Check sheet for the modelled part. Datum: model origin and axes. Units: mm. Coordinates: 2 decimals unless noted, no trailing zeros. Loops run counter-clockwise (first coordinate to the right, second up) from the corner with the lowest first, then second, coordinate; pieces in that order, holes last. Notation, with made-up numbers: (-32, 47) -> (14, 47) arc R7 ccw to (14, 53) -> close; hole circle Ø2 at (-26.5, 83). An arc over 180 degrees is marked (long way). Use one line per item in the form item = value.
from build123d import *

# Parameters (mm, degrees)
SKETCH1_R           = 11.25
SKETCH1_R_2         = 1.75
BOSS_EXTRUDE1_DEPTH = 3


with BuildPart() as part:
    # Sketch1 → Boss-Extrude1 (new body)
    with BuildSketch(Plane.XY):
        with BuildLine():
            Line((-125.662997175, -15.687527708), (-84.162997175, -15.687527708))
            Line((-84.162997175, -15.687527708), (-84.162997175, 25.812472292))
            Line((-84.162997175, 25.812472292), (-84.162997175, 30.812472292))
            Line((-84.162997175, 30.812472292), (-93.033440026, 55.812472292))
            Line((-93.033440026, 55.812472292), (-138.033440026, 55.812472292))
            Line((-138.033440026, 55.812472292), (-138.033440026, 54.312472292))
            ThreePointArc((-138.033440026, 54.312472292), (-126.533440026, 42.812472292), (-138.033440026, 31.312472292))
            Line((-138.033440026, 31.312472292), (-138.033440026, 30.812472292))
            Line((-138.033440026, 30.812472292), (-125.662997175, 30.812472292))
            Line((-125.662997175, 30.812472292), (-125.662997175, 25.812472292))
            Line((-125.662997175, 25.812472292), (-125.662997175, -15.687527708))
        make_face()
        with Locations((-108.033440026, 42.812472292)):
            Circle(SKETCH1_R, mode=Mode.SUBTRACT)
        with Locations((-89.412997175, 20.562472292)):
            Circle(SKETCH1_R_2, mode=Mode.SUBTRACT)
        with Locations((-120.412997175, 20.562472292)):
            Circle(SKETCH1_R_2, mode=Mode.SUBTRACT)
        with Locations((-120.412997175, -10.437527708)):
            Circle(SKETCH1_R_2, mode=Mode.SUBTRACT)
        with Locations((-89.412997175, -10.437527708)):
            Circle(SKETCH1_R_2, mode=Mode.SUBTRACT)
        with Locations((-122.733440026, 50.812472292)):
            Circle(SKETCH1_R_2, mode=Mode.SUBTRACT)
        with Locations((-122.733440026, 33.812472292)):
            Circle(SKETCH1_R_2, mode=Mode.SUBTRACT)
        with Locations((-92.733440026, 33.812472292)):
            Circle(SKETCH1_R_2, mode=Mode.SUBTRACT)
    extrude(amount=BOSS_EXTRUDE1_DEPTH)


solid = part.part
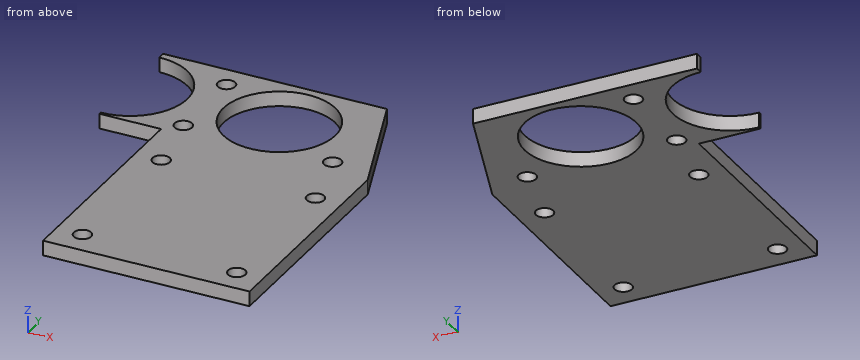
(1) Section check C-C, the plane z = 2.35. Give the number of separate pieces and of enclosed holes in the cut face, plus the area to 3 significant figures.
Established:
separate_pieces = 1
enclosed_holes = 8
area = 2,490 mm²
(2) Go/stop test with a flat-tipped pin: P1, Ø1, axis at y = 34, z = 2.5, coming from the +X side. Record where the tip stops, or that it passes through.
Established:
P1 = -85.12
(3) Section check A-A, the plane x = -105. Record the boundary of the cut face in (y, z), plus the area to 4 significant figures.
Established:
outline = (-15.69, 0) -> (31.98, 0) -> (31.98, 3) -> (-15.69, 3) -> close; (53.65, 0) -> (55.81, 0) -> (55.81, 3) -> (53.65, 3) -> close
area = 149.5 mm²
(4) Section check B-B, the plane y = 38.5. Record the boundary of the cut face in (x, z), plus the area to 3 significant figures.
Established:
outline = (-127.37, 0) -> (-118.42, 0) -> (-118.42, 3) -> (-127.37, 3) -> close; (-97.64, 0) -> (-86.89, 0) -> (-86.89, 3) -> (-97.64, 3) -> close
area = 59.1 mm²
(5) Scan lines: line 1 along X through (y, z) = (20.5, 0.85); line 2 along X through (y, z) = (-10, 1.4); line 3 along Y through (x, z) = (-119.5, 1.85). Record each from-to range of solid material in increasing order.
Established:
line_1 = -125.66 to -122.16, -118.66 to -91.16, -87.66 to -84.16
line_2 = -125.66 to -122.11, -118.72 to -91.11, -87.72 to -84.16
line_3 = -15.69 to -11.93, -8.94 to 19.07, 22.06 to 55.81
(6) Section check D-D, the plane y = 29.5. Record the boundary of the cut face in (x, z), plus the area to 4 significant figures.
Established:
outline = (-125.66, 0) -> (-84.16, 0) -> (-84.16, 3) -> (-125.66, 3) -> close
area = 124.5 mm²
